The listing builds one solid part. Answer for the finished solid, in the listing's coordinates (mm). A direction names the side the tool comes from. Round coordinates to 2 decimals unless told otherwise and drop trailing zeros. Loops run counter-clockwise (first coordinate to the right, second up) from the corner with the lowest first, then second, coordinate; pieces in that order, holes last. Notation, with made-up numbers: (-29.5, -24) - (-16.5, -24) arc R19 cw to (-16.5, -1) - close; hole circle Ø3 at (76.5, 0). An arc over 180 degrees is marked (long way). Write item = value, one per line. Start each with the question number.
1) Straight lines are drawn through the part: line 1 along X through (y, z) = (2.75, 24.5); line 2 along Z through (x, y) = (-4, 1); line 3 along X through (y, z) = (0.45, -40.6). For each, find the intervals that lie inside material, in ascending order.
2) Section C-C, the plane x = 24.17 is taken. Determine the outline of the cut face in (y, z).
3) Section B-B, the plane x = 45.5 is taken. Determine the outline of the cut face in (y, z), and give its area (4 significant figures).
4) Section D-D, the plane y = 2.75 is taken. Give the number of separate pieces and of enclosed holes in the cut face, and give its area (3 significant figures).
5) A tool of negligible diameter and unlimited length cuts with its end or side. For faces 1 (the flat face through (-8.299, 2.535, 45.453)), 2 (the flat face through (30, -2, 32)), 3 (the flat face through (-38, 0.5, 10)), from which of +Z, -Z, +X, -X, +Y, -Y can it reach the whole face along a straight path? Write none if from no direction.
6) For a pull along Z with two mould halves and no side action, classify faces 4 (the flat face through (-1, 0, -15)), 5 (the cylindrical face through (-63.59, 0.25, 11.07)) as released by +Z, released by -Z, zero draft, split by the parting line, or undercut.
7) Given pin 1 Ø2.5 at (x, z) = (24.17, -40.6) entering from +Y; pin 2 Ø4 at (x, z) = (25, -41.5) entering from -Y; pin 3 Ø6 at (x, z) = (61, 10.5) entering from +Y; pin 4 Ø0.6 at (y, z) = (-1, 31.5) entering from -X, each flat-ended and moving along its own axis, determine where each tip first touches the part or whether it passes through.
8) Section A-A, the plane z = -33.11 is taken. Determine the outline of the cut face in (x, y), and give its area (3 significant figures).
from build123d import *

# Parameters (mm, degrees)
SKETCH1_W           = 130
SKETCH1_H           = 125
BOSS_EXTRUDE1_DEPTH = 5
SKETCH2_R           = 1.75
SKETCH2_R_2         = 12.65
CUT_EXTRUDE1_DEPTH  = 10
SKETCH3_R           = 2.15
CUT_EXTRUDE2_DEPTH  = 10
SKETCH4_R           = 2.15
CUT_EXTRUDE3_DEPTH  = 10
BOSS_EXTRUDE2_DEPTH = 2
SKETCH6_R           = 2.65
CUT_EXTRUDE5_DEPTH  = 0.5
CUT_EXTRUDE7_DEPTH  = 91.444734507


with BuildPart() as part:
    # Sketch1 → Boss-Extrude1 (new body)
    with BuildSketch(Plane(origin=(0, 0, 0), x_dir=(1, 0, 0), z_dir=(0, 1, 0))):
        Rectangle(SKETCH1_W, SKETCH1_H)
    extrude(amount=BOSS_EXTRUDE1_DEPTH)

    # Sketch2 → Cut-Extrude1 (cut)
    with BuildSketch(Plane(origin=(0, 5, 0), x_dir=(1, 0, 0), z_dir=(0, 1, 0))):
        with Locations(Location((-61, -52.5, 0), (0, 0, 270))):
            Circle(SKETCH2_R)
        with Locations(Location((-36, -52.5, 0), (0, 0, 270))):
            Circle(SKETCH2_R)
        with Locations(Location((-36, -10.5, 0), (0, 0, 270))):
            Circle(SKETCH2_R)
        with Locations(Location((-61, -10.5, 0), (0, 0, 270))):
            Circle(SKETCH2_R)
        with Locations(Location((-45.5, -31.5, 0), (0, 0, 270))):
            Circle(SKETCH2_R_2)
    cut_extrude1 = extrude(amount=-CUT_EXTRUDE1_DEPTH, mode=Mode.SUBTRACT)

    # Mirror3: Cut-Extrude1 across plane
    add(cut_extrude1.mirror(Plane.ZY), mode=Mode.SUBTRACT)

    # Sketch3 → Cut-Extrude2 (cut)
    with BuildSketch(Plane(origin=(0, 5, 0), x_dir=(1, 0, 0), z_dir=(0, 1, 0))):
        with Locations(Location((-24.17, -42.03, 0), (0, 0, 270))):
            Circle(SKETCH3_R)
        with Locations(Location((24.17, -42.03, 0), (0, 0, 270))):
            Circle(SKETCH3_R)
        with Locations(Location((-8.73, 9.6, 0), (0, 0, 270))):
            Circle(SKETCH3_R)
        with Locations(Location((19.29, 9.6, 0), (0, 0, 270))):
            Circle(SKETCH3_R)
        with Locations(Location((-24.17, 33.11, 0), (0, 0, 270))):
            Circle(SKETCH3_R)
        with Locations(Location((24.17, 40.6, 0), (0, 0, 270))):
            Circle(SKETCH3_R)
    extrude(amount=-CUT_EXTRUDE2_DEPTH, mode=Mode.SUBTRACT)

    # Sketch4 → Cut-Extrude3 (cut)
    with BuildSketch(Plane(origin=(0, 5, 0), x_dir=(1, 0, 0), z_dir=(0, 1, 0))):
        with Locations(Location((0, 47.5, 0), (0, 0, 270))):
            Circle(SKETCH4_R)
        with Locations(Location((12.049810205, 55, 0), (0, 0, 270))):
            Circle(SKETCH4_R)
        with Locations(Location((-12.049810205, 55, 0), (0, 0, 270))):
            Circle(SKETCH4_R)
    extrude(amount=-CUT_EXTRUDE3_DEPTH, mode=Mode.SUBTRACT)

    # Sketch5 → Boss-Extrude2 (add)
    with BuildSketch(Plane.XZ):
        Polygon((-65, 58.7), (-65, 56.7), (-31.6, 56.7), (-31.6, 6.3), (-65, 6.3), (-65, 4.3), (-29.6, 4.3), (-29.6, 58.7), align=None)
    boss_extrude2 = extrude(amount=BOSS_EXTRUDE2_DEPTH)

    # Mirror6: Boss-Extrude2 across plane
    add(boss_extrude2.mirror(Plane.ZY))

    # Sketch6 → Cut-Extrude5 (cut)
    with BuildSketch(Plane.XZ):
        with Locations(Location((-8.73, -9.6, 0), (0, 0, 270))):
            Circle(SKETCH6_R)
        with Locations(Location((19.29, -9.6, 0), (0, 0, 270))):
            Circle(SKETCH6_R)
        with Locations(Location((-24.17, -33.11, 0), (0, 0, 270))):
            Circle(SKETCH6_R)
        with Locations(Location((24.17, -40.6, 0), (0, 0, 270))):
            Circle(SKETCH6_R)
        with Locations(Location((0, -47.5, 0), (0, 0, 270))):
            Circle(SKETCH6_R)
        with Locations(Location((-12.049810205, -55, 0), (0, 0, 270))):
            Circle(SKETCH6_R)
        with Locations(Location((12.049810205, -55, 0), (0, 0, 270))):
            Circle(SKETCH6_R)
        with Locations(Location((-61, 10.5, 0), (0, 0, 270))):
            Circle(SKETCH6_R)
        with Locations(Location((-36, 10.5, 0), (0, 0, 270))):
            Circle(SKETCH6_R)
        with Locations(Location((-36, 52.5, 0), (0, 0, 270))):
            Circle(SKETCH6_R)
        with Locations(Location((-61, 52.5, 0), (0, 0, 270))):
            Circle(SKETCH6_R)
        with Locations(Location((36, 52.5, 0), (0, 0, 270))):
            Circle(SKETCH6_R)
        with Locations(Location((36, 10.5, 0), (0, 0, 270))):
            Circle(SKETCH6_R)
        with Locations(Location((61, 10.5, 0), (0, 0, 270))):
            Circle(SKETCH6_R)
        with Locations(Location((61, 52.5, 0), (0, 0, 270))):
            Circle(SKETCH6_R)
        with Locations(Location((-24.17, 42.03, 0), (0, 0, 270))):
            Circle(SKETCH6_R)
        with Locations(Location((24.17, 42.03, 0), (0, 0, 270))):
            Circle(SKETCH6_R)
    extrude(amount=-CUT_EXTRUDE5_DEPTH, mode=Mode.SUBTRACT)

    # Sketch7 → Cut-Extrude7 (cut, through all)
    with BuildSketch(Plane(origin=(0, 5, 0), x_dir=(1, 0, 0), z_dir=(0, 1, 0))):
        Polygon((-3.163736655, -27.444416058), (-20.17, 0), (-20.17, -54.888832116), align=None)
        Polygon((17.332982786, 5.6), (-17.003730784, 5.6), (0.164626001, -22.10599967), align=None)
        Polygon((20.17, -54.888832116), (20.17, 0), (3.163736655, -27.444416058), align=None)
        Polygon((0.164626001, -31.79400033), (-17.003730784, -59.5), (17.332982786, -59.5), align=None)
    extrude(amount=-CUT_EXTRUDE7_DEPTH, mode=Mode.SUBTRACT)


solid = part.part
Geometry check:
q1.line_1 = -65 to -56.04, -34.96 to -20.17, -4.99 to 4.99, 20.17 to 34.96, 56.04 to 65
q1.line_2 = -62.5 to -5.6, 15.39 to 26.09, 28.79 to 38.51, 59.5 to 62.5
q1.line_3 = -65 to 21.52, 26.82 to 65
q2.outline = (0, -62.5) - (5, -62.5) - (5, -42.75) - (0.5, -42.75) - (0.5, -43.25) - (0, -43.25) - close; (0, -37.95) - (0.5, -37.95) - (0.5, -38.45) - (5, -38.45) - (5, 39.88) - (0.5, 39.88) - (0.5, 39.38) - (0, 39.38) - close; (0, 44.68) - (0.5, 44.68) - (0.5, 44.18) - (5, 44.18) - (5, 62.5) - (0, 62.5) - close
q3.outline = (-2, 4.3) - (0, 4.3) - (0, -62.5) - (5, -62.5) - (5, 18.85) - (0, 18.85) - (0, 6.3) - (-2, 6.3) - close; (-2, 56.7) - (0, 56.7) - (0, 44.15) - (5, 44.15) - (5, 62.5) - (0, 62.5) - (0, 58.7) - (-2, 58.7) - close
q3.area = 506.5 mm2
q4.separate_pieces = 1
q4.enclosed_holes = 23
q4.area = 13,200 mm2
q5.face_1 = +Y, -Y
q5.face_2 = +Z, -Z, +X, -X, -Y
q5.face_3 = -Y
q6.face_4 = zero draft
q6.face_5 = undercut
q7.pin_1 = through
q7.pin_2 = 0
q7.pin_3 = 5
q7.pin_4 = -31.6
q8.outline = (-65, 0) - (-26.82, 0) - (-26.82, 0.5) - (-26.32, 0.5) - (-26.32, 5) - (-65, 5) - close; (-22.02, 0.5) - (-21.52, 0.5) - (-21.52, 0) - (65, 0) - (65, 5) - (-22.02, 5) - close
q8.area = 628 mm2
